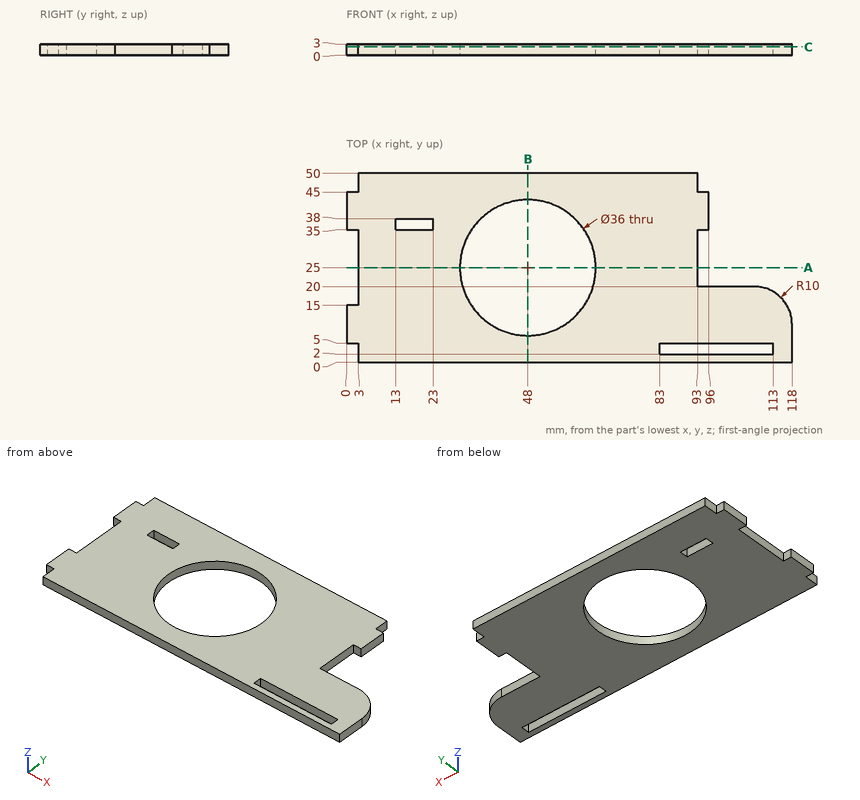
Design review of the part shown in the three views and the two pictorial views. Dimensions are in mm from the part's minimum x, y and z. Give positions to 0.01 mm unless a question says otherwise; leave off trailing zeros. Loops run counter-clockwise (first coordinate to the right, second up) from the corner with the lowest first, then second, coordinate; pieces in that order, holes last. Notation, with made-up numbers: M 85.5,60.5 L 93.5,60.5 A19 ccw 93.5,72.5 Z; hole C -2.75,65.25 d2. An arc over 180 degrees is marked long. Put each result on its own line as item: value. Start each with the question number.
(1) Wall thickness on L1, parallel to Y at x = 48, z = 1.1; L2, parallel to X at y = 37.5, z = 0.65; L3, parallel to Y at x = 31.5, z = 0.65: over which ranges is each line inside the solid? List them lowest first.
(2) Add section C-C, the plane z = 2.25. Write out the cut boundary in (x, y).
(3) Add section B-B, the plane x = 48. Write out the cut boundary in (y, z).
(4) For pin 1 (0.9 mm diameter, centred on x = 95, z = 2, fed in from +Y); pin 2 (0.9 mm diameter, centred on y = 47, z = 1, fed in from -X); pin 3 (1.5 mm diameter, centred on y = 38.5, z = 2, fed in from +X), all flat-tipped, find the tip position at first contact; note any pin that passes through.
(5) Add section A-A, the plane y = 25. Write out the cut boundary in (x, z), then the cut area to 3 significant figures.
Result:
1. L1: y = 0 to 7, 43 to 50
1. L2: x = 0 to 13, 23 to 35.05, 60.95 to 96
1. L3: y = 0 to 17.81, 32.19 to 50
2. outline: M 0,5 L 3,5 L 3,0 L 118,0 L 118,10 A10 ccw 108,20 L 93,20 L 93,35 L 96,35 L 96,45 L 93,45 L 93,50 L 3,50 L 3,45 L 0,45 L 0,35 L 3,35 L 3,15 L 0,15 Z; hole M 13,35 L 23,35 L 23,38 L 13,38 Z; hole C 48,25 d36; hole M 83,2 L 113,2 L 113,5 L 83,5 Z
3. outline: M 0,0 L 7,0 L 7,3 L 0,3 Z; M 43,0 L 50,0 L 50,3 L 43,3 Z
4. pin 1: stops at y = 45
4. pin 2: stops at x = 3
4. pin 3: stops at x = 96
5. outline: M 3,0 L 30,0 L 30,3 L 3,3 Z; M 66,0 L 93,0 L 93,3 L 66,3 Z
5. area: 162 mm^2
